from build123d import *
from OCP.BRepFilletAPI import BRepFilletAPI_MakeChamfer

# Parameters (mm, degrees)
BOSS_EXTRUDE1_DEPTH = 16.9
BOSS_EXTRUDE2_DEPTH = 13.5
BOSS_EXTRUDE3_DEPTH = 3.4
BOSS_EXTRUDE4_DEPTH = 13.5
CUT_EXTRUDE1_DEPTH  = 46.491242289
CHAMFER1_SIZE       = 2
CHAMFER1_SIZE2      = 1.154700538
CUT_EXTRUDE2_DEPTH  = 47.613443608
FILLET1_R           = 0.5
SKETCH10_W          = 25
SKETCH10_H          = 29.7
CUT_EXTRUDE3_DEPTH  = 47.613443644


with BuildPart() as part:
    # Sketch1 → Boss-Extrude1 (new body)
    with BuildSketch(Plane.XY):
        Polygon((-20, -13.85), (20, -13.85), (20, 13.85), (-20, 13.85), (-20, 14.85), (21, 14.85), (21, -14.85), (-20, -14.85), align=None)
    extrude(amount=BOSS_EXTRUDE1_DEPTH)

    # Sketch4 → Boss-Extrude2 (add)
    with BuildSketch(Plane(origin=(0, 0, 0), x_dir=(-1, 0, 0), z_dir=(0, 0, -1))):
        with BuildLine():
            Line((-21, 4.825), (-36, 4.825))
            ThreePointArc((-36, 4.825), (-38.610615349, 4.05774722), (-40.390970849, 2))
            Line((-40.390970849, 2), (-30.875, 2))
            Line((-30.875, 2), (-30.875, -2))
            Line((-30.875, -2), (-40.390970849, -2))
            ThreePointArc((-40.390970849, -2), (-38.610615349, -4.05774722), (-36, -4.825))
            Line((-36, -4.825), (-21, -4.825))
            Line((-21, -4.825), (-21, 4.825))
        make_face()
    extrude(amount=-BOSS_EXTRUDE2_DEPTH)

    # Sketch5 → Boss-Extrude3 (add)
    with BuildSketch(Plane.XY.offset(13.5)):
        with BuildLine():
            Line((21, 4.825), (21, -4.825))
            Line((21, -4.825), (36, -4.825))
            ThreePointArc((36, -4.825), (38.610615349, -4.05774722), (40.390970849, -2))
            ThreePointArc((40.390970849, -2), (40.825, 0), (40.390970849, 2))
            ThreePointArc((40.390970849, 2), (38.610615349, 4.05774722), (36, 4.825))
            Line((36, 4.825), (21, 4.825))
        make_face()
    extrude(amount=BOSS_EXTRUDE3_DEPTH)

    # Sketch8 → Boss-Extrude4 (add)
    with BuildSketch(Plane(origin=(0, 0, 0), x_dir=(-1, 0, 0), z_dir=(0, 0, -1))):
        with BuildLine():
            Line((-37.5, 2), (-40.390970849, 2))
            ThreePointArc((-40.390970849, 2), (-40.825, 0), (-40.390970849, -2))
            Line((-40.390970849, -2), (-37.5, -2))
            ThreePointArc((-37.5, -2), (-38.5, 0), (-37.5, 2))
        make_face()
        with BuildLine():
            Line((-34.5, 2), (-30.875, 2))
            Line((-30.875, 2), (-30.875, -2))
            Line((-30.875, -2), (-34.5, -2))
            ThreePointArc((-34.5, -2), (-33.5, 0), (-34.5, 2))
        make_face()
    extrude(amount=-BOSS_EXTRUDE4_DEPTH)

    # Sketch9 → Cut-Extrude1 (cut, through all)
    with BuildSketch(Plane(origin=(0, 0, 13.5), x_dir=(-1, 0, 0), z_dir=(0, 0, -1))):
        with BuildLine():
            Line((-37.5, -2), (-34.5, -2))
            ThreePointArc((-34.5, -2), (-33.5, 0), (-34.5, 2))
            Line((-34.5, 2), (-37.5, 2))
            ThreePointArc((-37.5, 2), (-38.5, 0), (-37.5, -2))
        make_face()
    extrude(amount=-CUT_EXTRUDE1_DEPTH, mode=Mode.SUBTRACT)

    # Chamfer1: one chamfer whose edges measure the first distance from different faces: ONE call of the kernel's chamfer builder (chamfer() names one face for all edges)
    chamfer1_edges_1 = [part.edges().sort_by_distance(p)[0] for p in [
        (36, 2, 0),
    ]]
    chamfer1_side_1 = [part.faces().sort_by_distance(p)[0] for p in [
        (36, 2, 8.45),
    ]]
    chamfer1_edges_2 = [part.edges().sort_by_distance(p)[0] for p in [
        (38.5, 0, 0),
    ]]
    chamfer1_side_2 = [part.faces().sort_by_distance(p)[0] for p in [
        (38.5, 0, 8.45),
    ]]
    chamfer1_edges_3 = [part.edges().sort_by_distance(p)[0] for p in [
        (36, -2, 0),
    ]]
    chamfer1_side_3 = [part.faces().sort_by_distance(p)[0] for p in [
        (36, -2, 8.45),
    ]]
    chamfer1_edges_4 = [part.edges().sort_by_distance(p)[0] for p in [
        (33.5, 0, 0),
    ]]
    chamfer1_side_4 = [part.faces().sort_by_distance(p)[0] for p in [
        (33.5, 0, 8.45),
    ]]
    chamfer1 = BRepFilletAPI_MakeChamfer(part.part.solid().wrapped)
    for e in chamfer1_edges_1:
        chamfer1.Add(CHAMFER1_SIZE, CHAMFER1_SIZE2, e.wrapped, chamfer1_side_1[0].wrapped)  # the first distance lies on this face
    for e in chamfer1_edges_2:
        chamfer1.Add(CHAMFER1_SIZE, CHAMFER1_SIZE2, e.wrapped, chamfer1_side_2[0].wrapped)  # the first distance lies on this face
    for e in chamfer1_edges_3:
        chamfer1.Add(CHAMFER1_SIZE, CHAMFER1_SIZE2, e.wrapped, chamfer1_side_3[0].wrapped)  # the first distance lies on this face
    for e in chamfer1_edges_4:
        chamfer1.Add(CHAMFER1_SIZE, CHAMFER1_SIZE2, e.wrapped, chamfer1_side_4[0].wrapped)  # the first distance lies on this face
    add(Compound.cast(chamfer1.Shape()), mode=Mode.REPLACE)

    # Sketch11 → Cut-Extrude2 (cut, through all)
    with BuildSketch(Plane(origin=(0, 0, 0), x_dir=(-1, 0, 0), z_dir=(0, 0, -1))):
        with BuildLine():
            Line((-34.483424911, 2.05), (-37.516575089, 2.05))
            ThreePointArc((-37.516575089, 2.05), (-38.55, 0), (-37.516575089, -2.05))
            Line((-37.516575089, -2.05), (-34.483424911, -2.05))
            ThreePointArc((-34.483424911, -2.05), (-33.45, 0), (-34.483424911, 2.05))
        make_face()
    extrude(amount=-CUT_EXTRUDE2_DEPTH, mode=Mode.SUBTRACT)

    # Fillet1
    fillet1_edges = [part.edges().sort_by_distance(p)[0] for p in [
        (-20, 14.85, 8.45),
        (21, 14.85, 8.45),
        (21, -14.85, 8.45),
        (-20, -14.85, 8.45),
    ]]
    fillet(fillet1_edges, radius=FILLET1_R)

    # Sketch10 → Cut-Extrude3 (cut, through all)
    with BuildSketch(Plane(origin=(0, 0, 0), x_dir=(-1, 0, 0), z_dir=(0, 0, -1))):
        with Locations((7.5, 0)):
            Rectangle(SKETCH10_W, SKETCH10_H)
    extrude(amount=-CUT_EXTRUDE3_DEPTH, mode=Mode.SUBTRACT)


solid = part.part
Can you work these out from the model? Positions are in its coordinate system, mm. A direction names the side the tool comes from. Give positions to 0.01 mm unless a question says otherwise; leave off trailing zeros. Write each loop counter-clockwise with the first axis right and the second up, starting at its lowest first coordinate (ties: lowest second). Pieces come first, ordered by that corner, then holes. Notation, with made-up numbers: M -33,58.25 L 15,58.25 A15 cw 15,67.25 Z; hole C 3.5,2.25 d8. An arc over 180 degrees is marked long. Answer in a Markdown table with one row per item. Add a question column.
Item 1: We'd pull the mould along X, two halves only. Please class faces 1 (the flat face through (36, 2.05, 9)), 2 (the flat face through (13, -14.85, 8)), 3 (the flat face through (5, 14, 8)): released by +X, released by -X, zero draft, split by the parting line, or undercut.
Item 2: On a 3-axis mill with a long thin cutter (end or side, diameter ignored), from which of +Z, -Z, +X, -X, +Y, -Y can I reach the whole of each face in a straight line? I mean faces 4 (the flat face through (12, -13.85, 8)), 5 (the conical face through (33.013, -0.044, 1.156)), 6 (the flat face through (28, -4.825, 8)), 7 (the cylindrical face through (33.45, -0.03, 9.3)). Say none if no direction works.
Item 3: For pin 1 Ø2 at (x, z) = (26, 9) entering from -Y (3 decimals); pin 2 Ø7.5 at (y, z) = (-11, 6.5) entering from +X; pin 3 Ø1 at (y, z) = (8.5, 9.5) entering from -X, each with a flat end and sliding along its axis, tell me the tip position at first contact or that it passes through.
Item 4: Imagine slicing it at A-A, the plane y = 0. Write out the boundary of the cut face in (x, z) (3 decimals).
Item 5: Imagine slicing it at D-D, the plane x = 26.5. Write out the boundary of the cut face in (y, z) (3 decimals).
Item 6: Imagine slicing it at B-B, the plane x = 13.5. Write out the boundary of the cut face in (y, z).
Item 7: Please list where these lines run through material, in increasing order: L1, parallel to Y at x = 12.5, z = 10; L2, parallel to X at y = -10.75, z = 6; L3, parallel to X at y = -2, z = 1.
Item 8: Imagine slicing it at C-C, the plane z = 11. Write out the boundary of the cut face in (x, y) (3 decimals).
Evaluation:
| question | item | result |
|---|---|---|
| 1 | face 1 | undercut |
| 1 | face 2 | zero draft |
| 1 | face 3 | released by -X |
| 2 | face 4 | +Z, -Z, -X |
| 2 | face 5 | -Z |
| 2 | face 6 | +Z, -Z, +X, -Y |
| 2 | face 7 | +Z, -Z |
| 3 | pin 1 | stops at y = -4.825 |
| 3 | pin 2 | stops at x = 21 |
| 3 | pin 3 | stops at x = 20 |
| 4 | outline | M 20,0 L 32.345,0 L 33.45,1.913 L 33.45,16.9 L 20,16.9 Z; M 38.55,1.913 L 39.655,0 L 40.825,0 L 40.825,16.9 L 38.55,16.9 Z |
| 5 | outline | M -4.825,0 L 4.825,0 L 4.825,16.9 L -4.825,16.9 Z |
| 6 | outline | M -14.85,0 L -13.85,0 L -13.85,16.9 L -14.85,16.9 Z; M 13.85,0 L 14.85,0 L 14.85,16.9 L 13.85,16.9 Z |
| 7 | L1 | y = -14.85 to -13.85, 13.85 to 14.85 |
| 7 | L2 | x = 20 to 21 |
| 7 | L3 | x = 20 to 33.66, 38.34 to 40.39 |
| 8 | outline | M 5,-14.85 L 20.5,-14.85 A0.5 ccw 21,-14.35 L 21,-4.825 L 36,-4.825 A4.825 ccw 36,4.825 L 21,4.825 L 21,14.35 A0.5 ccw 20.5,14.85 L 5,14.85 L 5,13.85 L 20,13.85 L 20,-13.85 L 5,-13.85 Z; hole M 34.483,-2.05 L 37.517,-2.05 A2.55 ccw 37.517,2.05 L 34.483,2.05 A2.55 ccw Z |
